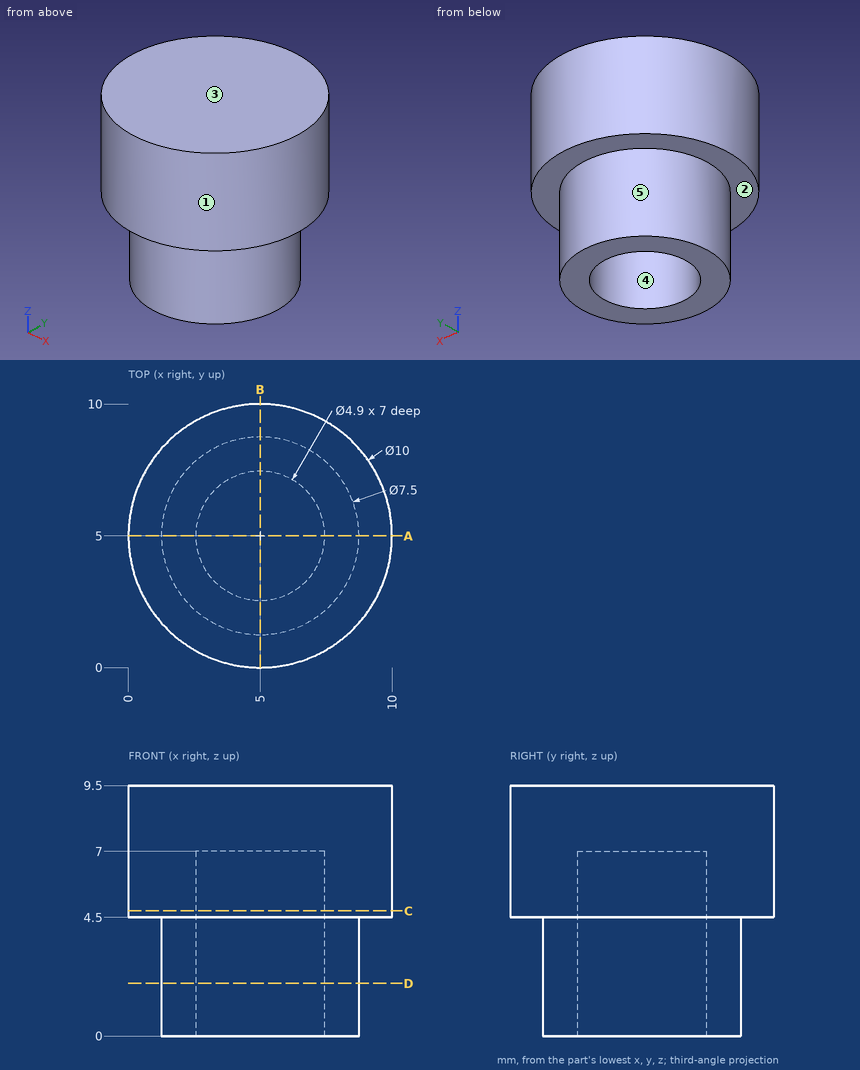
Check sheet for the drawn part. Datum: minimum x, y, z corner. Units: mm. A direction names the side the tool comes from. Round coordinates to 2 decimals unless told otherwise and drop trailing zeros. Order: outer loops, then holes, each group sorted by start corner. A loop starts at its lowest first (then second) coordinate and runs counter-clockwise, first axis right, second up. Notation, with made-up numbers: (89, -2) - (147, -2) arc R7 cw to (147, 11) - close; hole circle Ø4 at (33, 88.5). An arc over 180 degrees is marked (long way). Use a Markdown table: item, result. Add a question column.
(1) Release check for a two-part mould opening along Y. For the marked faces 3, 4 and 5 record: pulls with the +Y half, pulls with the -Y half, needs draft (parallel to the pull), parting line crosses it, or undercut.
(2) Material ranges on line 1 along Y through (x, z) = (5, 3.5); line 2 along Z through (x, y) = (9.5, 6); line 3 along X through (y, z) = (3.25, 3.75), recorded low to high. Write a range as [from, to].
(3) Depth check by flat-ended pin: pin 1 (2 mm diameter, centred on y = 7, z = 7.5, fed in from +X); pin 2 (1.5 mm diameter, centred on x = 6.5, z = 4, fed in from +Y); pin 3 (1 mm diameter, centred on x = 8.5, y = 7.5, fed in from -Z). Enter the tip coordinate at first touch or a pass-through.
(4) Sectioned sample at A-A, the plane y = 5. Enter the section's corners in (x, z), and give its area (4 significant figures).
(5) Sectioned sample at C-C, the plane z = 4.75. Enter the section's corners in (x, y), and give its area (3 significant figures).
(6) Tool access check on the marked faces 1 and 2. Record the directions out of +Z, -Z, +X, -X, +Y, -Y that give a thin tool (end or side, any length) a straight path to the whole face; none if there is none.
(7) Sectioned sample at D-D, the plane z = 2. Enter the section's corners in (x, y), and give its area (3 significant figures).
Answers below:
| question | item | result |
|---|---|---|
| 1 | face 3 | needs draft |
| 1 | face 4 | undercut |
| 1 | face 5 | parting line crosses it |
| 2 | line 1 | [1.25, 2.55], [7.45, 8.75] |
| 2 | line 2 | [4.5, 9.5] |
| 2 | line 3 | [1.68, 3.29], [6.71, 8.32] |
| 3 | pin 1 | x = 9.9 |
| 3 | pin 2 | y = 9.91 |
| 3 | pin 3 | z = 4.5 |
| 4 | outline | (0, 4.5) - (1.25, 4.5) - (1.25, 0) - (2.55, 0) - (2.55, 7) - (7.45, 7) - (7.45, 0) - (8.75, 0) - (8.75, 4.5) - (10, 4.5) - (10, 9.5) - (0, 9.5) - close |
| 4 | area | 49.45 mm² |
| 5 | outline | circle Ø10 at (5, 5); hole circle Ø4.9 at (5, 5) |
| 5 | area | 59.7 mm² |
| 6 | face 1 | +Z, -Z |
| 6 | face 2 | -Z |
| 7 | outline | circle Ø7.5 at (5, 5); hole circle Ø4.9 at (5, 5) |
| 7 | area | 25.3 mm² |
